Here's how the part is built. I have some questions about the finished solid (model axes, mm). A direction names the side the tool comes from. Give positions to 0.01 mm unless a question says otherwise; leave off trailing zeros. Write each loop counter-clockwise with the first axis right and the second up, starting at its lowest first coordinate (ties: lowest second). Pieces come first, ordered by that corner, then holes. Notation, with made-up numbers: (78, 9) - (121, 9) arc R18 ccw to (121, 34) - close; hole circle Ø3 at (61, 65). An arc over 180 degrees is marked (long way). Write each question's results on one line, items separated by ' | '. Start each with the question number.
Item 1: Please list where these lines run through material, in increasing order: line 1 along X through (y, z) = (-10, 241.5); line 2 along Z through (x, y) = (300, -3.25); line 3 along X through (y, z) = (-2.5, 109.5).
Item 2: Will these pins go through, and if not, where does the flat tip stop? P1, Ø2, axis at x = 327, y = -7.5, coming from the +Z side; P2, Ø4, axis at x = 78.5, z = -116.5, coming from the +Y side; P3, Ø3.5, axis at y = -7, z = 253, coming from the +X side; P4, Ø6, axis at y = -10, z = -92.5, coming from the -X side.
Item 3: We'd pull the mould along Z, two halves only. Please class faces 1 (the flat face through (162.123, -5.916, 37.339)), 2 (the cylindrical face through (404.54, -5.92, -186.19)), 3 (the flat face through (-129.944, -5.916, 44.643)), 4 (the flat face through (9, -12, -30)): +Z half, -Z half, draft (parallel to the pull), parting line (faces both ways), or undercut.
Item 4: Suppose I cut it at B-B on y = -6.5. List the corners of the cut face in (x, z) for me, then the cut area to 3 significant figures.
Item 5: Suppose I cut it at A-A on x = -125. List the corners of the cut face in (y, z) for me, then the cut area to 3 significant figures.
Item 6: Suppose I cut it at C-C on z = 92. List the corners of the cut face in (x, y) for me, then the cut area to 3 significant figures.
Item 7: Which directions (+Z, -Z, +X, -X, +Y, -Y) give clear straight access to the entire face, cutting with the end or side of a thin tool? Please do faces 5 (the flat face through (-119.16, -5.92, 225.82)), 6 (the cylindrical face through (118.279, -5.916, 193.664)).
Item 8: Suppose I cut it at D-D on x = 320. List the corners of the cut face in (y, z) for me, then the cut area to 3 significant figures.
```python
from build123d import *

# Parameters (mm, degrees)
F1_DEPTH = 12


with BuildPart() as f1:
    # F0 (on Front) → F1 (new body)
    with BuildSketch(Plane.XZ):
        with BuildLine():
            Line((-385.239591, -216.748114), (-385.239591, -247.767903))
            Line((-385.239591, -247.767903), (414.760409, -247.767903))
            Line((414.760409, -247.767903), (414.760409, -216.748114))
            ThreePointArc((414.760409, -216.748114), (404.262759, -185.823034), (377.108417, -167.679082))
            Line((377.108417, -167.679082), (263.722384, -137.297386))
            ThreePointArc((263.722384, -137.297386), (228.788625, -118.13207), (206.651561, -85.001612))
            Line((206.651561, -85.001612), (116.330324, 163.153948))
            ThreePointArc((116.330324, 163.153948), (118.486024, 194.059957), (142.889403, 213.146694))
            Line((142.889403, 213.146694), (164.289631, 218.498353))
            Line((164.289631, 218.498353), (164.289631, 302.232097))
            Line((164.289631, 302.232097), (-134.768812, 302.232097))
            Line((-134.768812, 302.232097), (-134.768812, 233.465457))
            Line((-134.768812, 233.465457), (-103.102214, 217.953577))
            ThreePointArc((-103.102214, 217.953577), (-84.524765, 197.980438), (-84.060364, 170.70715))
            Line((-84.060364, 170.70715), (-177.130742, -85.001612))
            ThreePointArc((-177.130742, -85.001612), (-199.267807, -118.13207), (-234.201565, -137.297386))
            Line((-234.201565, -137.297386), (-347.587598, -167.679082))
            ThreePointArc((-347.587598, -167.679082), (-374.74194, -185.823034), (-385.239591, -216.748114))
        make_face()
    extrude(amount=F1_DEPTH)


solid = f1.part
```
Checked values:
1) line 1: x = -134.77 to 164.29 | line 2: z = -247.77 to -147.02 | line 3: x = -106.34 to 135.86
2) P1: stops at z = -153.98 | P2: stops at y = 0 | P3: stops at x = 164.29 | P4: stops at x = -181.79
3) face 1: undercut | face 2: +Z half | face 3: undercut | face 4: draft
4) outline: (-385.24, -247.77) - (414.76, -247.77) - (414.76, -216.75) arc R50.8 ccw to (377.11, -167.68) - (263.72, -137.3) arc R83.82 cw to (206.65, -85) - (116.33, 163.15) arc R38.1 cw to (142.89, 213.15) - (164.29, 218.5) - (164.29, 302.23) - (-134.77, 302.23) - (-134.77, 233.47) - (-103.1, 217.95) arc R38.1 cw to (-84.06, 170.71) - (-177.13, -85) arc R83.82 cw to (-234.2, -137.3) - (-347.59, -167.68) arc R50.8 ccw to (-385.24, -216.75) - close | area: 213,000 mm^2
5) outline: (-12, -247.77) - (0, -247.77) - (0, 58.23) - (-12, 58.23) - close; (-12, 228.68) - (0, 228.68) - (0, 302.23) - (-12, 302.23) - close | area: 4,550 mm^2
6) outline: (-112.71, -12) - (142.23, -12) - (142.23, 0) - (-112.71, 0) - close | area: 3,060 mm^2
7) face 5: -X, +Y, -Y | face 6: +X, +Y, -Y
8) outline: (-12, -247.77) - (0, -247.77) - (0, -152.38) - (-12, -152.38) - close | area: 1,140 mm^2
